from build123d import *

# Parameters (mm, degrees)
F0_W     = 38
F0_H     = 55
F0_W_2   = 25
F0_H_2   = 6.5
F0_W_3   = 7
F0_H_3   = 18
F1_DEPTH = 2.5
F2_R     = 15
F3_R     = 5
F4_R     = 3
F5_W     = 33
F5_H     = 3
F6_DEPTH = 3.5
F7_R     = 0.4
F8_R     = 0.9


with BuildPart() as f1:
    # F0 (on Front) → F1 (new body)
    with BuildSketch(Plane.XZ):
        with Locations((0, 27.5)):
            Rectangle(F0_W, F0_H)
        with Locations((0, 13.25)):
            Rectangle(F0_W_2, F0_H_2, mode=Mode.SUBTRACT)
        with Locations((0, 40.968925)):
            Rectangle(F0_W_3, F0_H_3, mode=Mode.SUBTRACT)
    extrude(amount=F1_DEPTH)

    # F2
    f2_edges = [f1.edges().sort_by_distance(p)[0] for p in [
        (-19, -1.25, 55),
        (19, -1.25, 55),
    ]]
    fillet(f2_edges, radius=F2_R)

    # F3
    f3_edges = [f1.edges().sort_by_distance(p)[0] for p in [
        (-19, -1.25, 0),
        (19, -1.25, 0),
    ]]
    fillet(f3_edges, radius=F3_R)

    # F4
    f4_edges = [f1.edges().sort_by_distance(p)[0] for p in [
        (-12.5, -1.25, 10),
        (12.5, -1.25, 10),
        (12.5, -1.25, 16.5),
        (-12.5, -1.25, 16.5),
        (-3.5, -1.25, 49.968925),
        (-3.5, -1.25, 31.968925),
        (3.5, -1.25, 31.968925),
        (3.5, -1.25, 49.968925),
    ]]
    fillet(f4_edges, radius=F4_R)

    # F5 (on face) → F6 (join)
    with BuildSketch(Plane(origin=(0, 0, 0), x_dir=(-1, 0, 0), z_dir=(0, 1, 0))):
        with Locations((0, 25.3)):
            Rectangle(F5_W, F5_H)
    extrude(amount=F6_DEPTH)

    # F7
    f7_edges = [f1.edges().sort_by_distance(p)[0] for p in [
        (19, 0, 22.5),
    ]]
    fillet(f7_edges, radius=F7_R)

    # F8
    f8_edges = [f1.edges().sort_by_distance(p)[0] for p in [
        (19, -2.5, 22.5),
    ]]
    fillet(f8_edges, radius=F8_R)


solid = f1.part
The listing builds one solid part. Answer for the finished solid, in the listing's coordinates (mm). A direction names the side the tool comes from. Coordinates: 2 decimals unless noted, no trailing zeros. Loops run counter-clockwise (first coordinate to the right, second up) from the corner with the lowest first, then second, coordinate; pieces in that order, holes last. Notation, with made-up numbers: M -19.5,70.5 L 38.5,70.5 A29 cw 38.5,108.5 Z; hole C 20,49.5 d6. An arc over 180 degrees is marked long. Answer in a Markdown table with one row per item.
1) Find the intervals of material crossed by probe 1 along Z at (x, y) = (-1, -0.25); probe 2 along Y at (x, z) = (-16.5, 38); probe 3 along Z at (x, y) = (-5, -0.1), in increasing order.
Answers below:
| item | result |
|---|---|
| probe 1 | 0.03 to 10, 16.5 to 32.01, 49.93 to 54.97 |
| probe 2 | -2.5 to 0 |
| probe 3 | 0.14 to 10, 16.5 to 54.83 |
2) Given pin 1 (0.9 mm diameter, centred on y = 2.5, z = 25.5, fed in from -X); pin 2 (0.9 mm diameter, centred on y = 2.5, z = 24.5, fed in from +X); pin 3 (1.5 mm diameter, centred on x = 0, y = 1, fed in from +Z), each flat-ended and moving along its own axis, determine where each tip first touches the part or whether it passes through.
Answers below:
| item | result |
|---|---|
| pin 1 | x = -16.5 |
| pin 2 | x = 16.5 |
| pin 3 | z = 26.8 |
3) Determine the mould class of faces 4 (the flat face through (16.5, 2, 25)), 5 (the flat face through (3.5, -1, 41)), 6 (the flat face through (0, -1, 0)) for opening direction Z: released by +Z, released by -Z, zero draft, split by the parting line, or undercut.
Answers below:
| item | result |
|---|---|
| face 4 | zero draft |
| face 5 | undercut |
| face 6 | released by -Z |
4) Find section B-B (y = -1). Determine the outline of the cut face in (x, z), then the cut area to 3 significant figures.
Answers below:
| item | result |
|---|---|
| outline | M -19,5 A5 ccw -14,0 L 14,0 A5 ccw 19,5 L 19,40 A15 ccw 4,55 L -4,55 A15 ccw -19,40 Z; hole M -12.5,13 A3 ccw -9.5,10 L 9.5,10 A3 ccw 12.5,13 L 12.5,13.5 A3 ccw 9.5,16.5 L -9.5,16.5 A3 ccw -12.5,13.5 Z; hole M -3.5,34.97 A3 ccw -0.5,31.97 L 0.5,31.97 A3 ccw 3.5,34.97 L 3.5,46.97 A3 ccw 0.5,49.97 L -0.5,49.97 A3 ccw -3.5,46.97 Z |
| area | 1,710 mm^2 |
5) Which of the six approach directions +Z, -Z, +X, -X, +Y, -Y give full straight-line access (tool end or side, diameter ignored) to faces 1 (the flat face through (0, 2, 23.8)), 2 (the flat face through (-16.5, 2, 25)), 3 (the cylindrical face through (11.6, -1.27, 10.86))?
Answers below:
| item | result |
|---|---|
| face 1 | -Z, +X, -X, +Y |
| face 2 | +Z, -Z, -X, +Y |
| face 3 | +Y, -Y |
6) Find section D-D (z = 31). Determine the outline of the cut face in (x, y).
Answers below:
| item | result |
|---|---|
| outline | M -19,-1.6 A0.9 ccw -18.1,-2.5 L 18.1,-2.5 A0.9 ccw 19,-1.6 L 19,-0.4 A0.4 ccw 18.6,0 L -18.6,0 A0.4 ccw -19,-0.4 Z |
7) Find section A-A (x = 2.5). Determine the outline of the cut face in (y, z) (3 decimals), then the cut area to 3 significant figures.
Answers below:
| item | result |
|---|---|
| outline | M -2.5,0.9 A0.9 ccw -1.6,0 L -0.4,0 A0.4 ccw 0,0.4 L 0,10 L -2.5,10 Z; M -2.5,16.5 L 0,16.5 L 0,23.8 L 3.5,23.8 L 3.5,26.8 L 0,26.8 L 0,32.733 L -2.5,32.733 Z; M -2.5,49.205 L 0,49.205 L 0,54.6 A0.4 ccw -0.4,55 L -1.6,55 A0.9 ccw -2.5,54.1 Z |
| area | 90.2 mm^2 |
8) Find section C-C (z = 12). Determine the outline of the cut face in (x, y).
Answers below:
| item | result |
|---|---|
| outline | M -19,-1.6 A0.9 ccw -18.1,-2.5 L -12.33,-2.5 L -12.33,0 L -18.6,0 A0.4 ccw -19,-0.4 Z; M 12.33,-2.5 L 18.1,-2.5 A0.9 ccw 19,-1.6 L 19,-0.4 A0.4 ccw 18.6,0 L 12.33,0 Z |
